Autodesk Inventor part; units mm, degrees
ref_plane "YZ Plane" through (0, 0, 0) normal (1, 0, 0) x (0, 1, 0)
ref_plane "XZ Plane" through (0, 0, 0) normal (0, 1, 0) x (-1, 0, 0)
ref_plane "XY Plane" through (0, 0, 0) normal (0, 0, 1) x (1, 0, 0)
sketch "Sketch1" plane through (0, 0, 0) normal (0, 1, 0) x (-1, 0, 0)
  line L0 (0, 0) -> (57.15, 0)
  line L1 (57.15, 0) -> (57.15, -87.63)
  line L2 (57.15, -87.63) -> (0, -87.63)
  line L3 (0, -87.63) -> (0, 0)
  line L4 (59.69, -90.17) -> (59.69, 2.54)
  line L5 (59.69, 2.54) -> (-2.54, 2.54)
  line L6 (-2.54, 2.54) -> (-2.54, -90.17)
  line L7 (-2.54, -90.17) -> (59.69, -90.17)
  dimension "d0" = 57.15
  dimension "d1" = 87.63
  dimension "d2" = 2.54
extrude "Extrusion1" add sketch "Sketch1" along normal blind 6.35 contours L0 L1 L2 L3
extrude "Extrusion2" add sketch "Sketch1" along normal blind 2.54
properties part number "LCD"
Verification items for the finished model (mm, model axes). A direction names the side the tool comes from. Coordinates: 2 decimals unless noted, no trailing zeros. Loops run counter-clockwise (first coordinate to the right, second up) from the corner with the lowest first, then second, coordinate; pieces in that order, holes last. Notation, with made-up numbers: (20, -1.75) -> (24, -1.75) arc R22 ccw to (24, 10.25) -> close; hole circle Ø4 at (61.5, 30.25). An arc over 180 degrees is marked (long way). Answer as a JSON object with one key per item and string values. Group by question number.
Item 1: Sectioned sample at C-C on y = 5. Record the boundary of the cut face in (x, z).
Item 2: Sectioned sample at A-A on z = -32.5. Record the boundary of the cut face in (x, y), plus the area to 3 significant figures.
Item 3: Scan lines: probe 1 along Z at (x, y) = (-16.5, 4.5); probe 2 along X at (y, z) = (3, -85.5). Record each from-to range of solid material in increasing order.
Item 4: Depth check by flat-ended pin: pin 1 (1.9 mm diameter, centred on y = 4, z = -39, fed in from +X); pin 2 (1.9 mm diameter, centred on x = -32, y = 4, fed in from +Z); pin 3 (1.9 mm diameter, centred on y = 4, z = -47, fed in from -X). Enter the tip coordinate at first touch or a pass-through.
Item 5: Tool access check on faces 1 (the flat face through (-57.15, 4, -43)), 2 (the flat face through (-28, 4, 0)), 3 (the flat face through (0, 4, -44)). Record the directions out of +Z, -Z, +X, -X, +Y, -Y that give a thin tool (end or side, any length) a straight path to the whole face; none if there is none.
Item 6: Sectioned sample at B-B on x = -12.5. Record the boundary of the cut face in (y, z), plus the area to 3 significant figures.
Evaluation:
{
 "1": {"outline": "(-57.15, -87.63) -> (0, -87.63) -> (0, 0) -> (-57.15, 0) -> close"},
 "2": {"outline": "(-59.69, 0) -> (2.54, 0) -> (2.54, 2.54) -> (0, 2.54) -> (0, 6.35) -> (-57.15, 6.35) -> (-57.15, 2.54) -> (-59.69, 2.54) -> close", "area": "376 mm²"},
 "3": {"probe 1": "z = -87.63 to 0", "probe 2": "x = -57.15 to 0"},
 "4": {"pin 1": "stops at x = 0", "pin 2": "stops at z = 0", "pin 3": "stops at x = -57.15"},
 "5": {"face 1": "+Z, -Z, -X, +Y", "face 2": "+Z, +X, -X, +Y", "face 3": "+Z, -Z, +X, +Y"},
 "6": {"outline": "(0, -90.17) -> (2.54, -90.17) -> (2.54, -87.63) -> (6.35, -87.63) -> (6.35, 0) -> (2.54, 0) -> (2.54, 2.54) -> (0, 2.54) -> close", "area": "569 mm²"}
}
